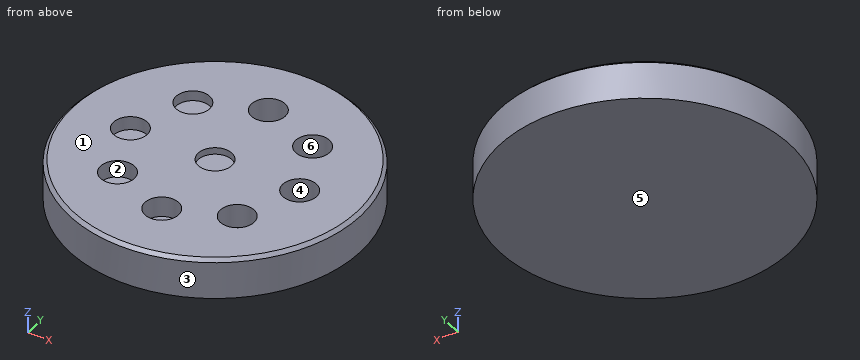
Autodesk Inventor part; units mm, degrees
ref_plane "YZ Plane" through (0, 0, 0) normal (1, 0, 0) x (0, 1, 0)
ref_plane "XZ Plane" through (0, 0, 0) normal (0, 1, 0) x (-1, 0, 0)
ref_plane "XY Plane" through (0, 0, 0) normal (0, 0, 1) x (1, 0, 0)
sketch "Sketch1" plane through (0, 0, 0) normal (0, 0, 1) x (1, 0, 0)
  circle A0 centre (0, 0) radius 43
  circle A1 centre (0, 0) radius 5
  circle A2 centre (0, 25) radius 5
  circle A3 centre (-17.6777, 17.6777) radius 5
  circle A4 centre (-25, 0) radius 5
  circle A5 centre (-17.6777, -17.6777) radius 5
  circle A6 centre (0, -25) radius 5
  circle A7 centre (17.6777, -17.6777) radius 5
  circle A8 centre (25, 0) radius 5
  circle A9 centre (17.6777, 17.6777) radius 5
  dimension "diameter" = 10
  dimension "d2" = 10
  dimension "d5" = 360
  dimension "d7" = 25
  dimension "d28" = 86
extrude "Extrusion1" add sketch "Sketch1" along normal blind 12
extrude "Extrusion2" add sketch "Sketch1" along normal blind 2 contours A2
extrude "Extrusion3" add sketch "Sketch1" along normal blind 3 contours A9
extrude "Extrusion4" add sketch "Sketch1" along normal blind 4 contours A8
extrude "Extrusion5" add sketch "Sketch1" along normal blind 5 contours A7
extrude "Extrusion6" add sketch "Sketch1" along normal blind 6 contours A6
extrude "Extrusion7" add sketch "Sketch1" along normal blind 7 contours A5
extrude "Extrusion8" add sketch "Sketch1" along normal blind 8 contours A4
extrude "Extrusion9" add sketch "Sketch1" along normal blind 9 contours A3
extrude "Extrusion10" add sketch "Sketch1" along normal blind 10 contours A1
sketch "Sketch2" plane through (0, 0, 12) normal (0, 0, 1) x (1, 0, 0)
  line L0 (-5.8774, 39.105) -> (5.7366, 39.105) construction
  line L1 (5.7366, 39.105) -> (5.7366, 35.936) construction
  line L2 (5.7366, 35.936) -> (-5.8774, 35.936) construction
  line L3 (-5.8774, 35.936) -> (-5.8774, 39.105) construction
  point P0 (0, 0)
emboss "Emboss1" [suppressed]
chamfer "Chamfer1" distance 1 angle 45 1 edges at (-43, 0, 12)
equation "\"d2\" = diameter"
properties part number "Diameter_10mm"
Can you work these out from the model? Positions are in its coordinate system, mm. Face numbers are marked on the shaded views. A direction names the side the tool comes from. Give positions to 0.01 mm unless a question says otherwise; leave off trailing zeros. Loops run counter-clockwise (first coordinate to the right, second up) from the corner with the lowest first, then second, coordinate; pieces in that order, holes last. Notation, with made-up numbers: M -2,54 L 43,54 A24 cw 43,67 Z; hole C 32.5,-31 d2. An arc over 180 degrees is marked long. One line per item, written item: value.
(1) Suppose I cut it at A-A on x = 0. List the corners of the cut face in (y, z) for me.
Returned:
outline: M -43,0 L 43,0 L 43,11 L 42,12 L 30,12 L 30,2 L 20,2 L 20,12 L 5,12 L 5,10 L -5,10 L -5,12 L -20,12 L -20,6 L -30,6 L -30,12 L -42,12 L -43,11 Z
(2) Suppose I cut it at B-B on y = 0. List the corners of the cut face in (x, z) for me.
Returned:
outline: M -43,0 L 43,0 L 43,11 L 42,12 L 30,12 L 30,4 L 20,4 L 20,12 L 5,12 L 5,10 L -5,10 L -5,12 L -20,12 L -20,8 L -30,8 L -30,12 L -42,12 L -43,11 Z
(3) I need wall thicknesses on line 1 (Y direction, x = 0, z = 5.75); line 2 (Y direction, x = 15, z = 7.75); line 3 (Y direction, x = 0, z = 11.1). Which ranges of each line are inside material? Lowest first, please.
Returned:
line 1: -43 to 20, 30 to 43
line 2: -40.3 to -21.9, -13.46 to 13.46, 21.9 to 40.3
line 3: -42.9 to -30, -20 to -5, 5 to 20, 30 to 42.9
(4) Which directions (+Z, -Z, +X, -X, +Y, -Y) give clear straight access to the entire face, cutting with the end or side of a thin tool? Please do the marked faces 5 and 6.
Returned:
face 5: -Z, +X, -X, +Y, -Y
face 6: +Z
(5) Will these pins go through, and if not, where does the flat tip stop? pin 1 (1 mm diameter, centred on y = 24.5, z = 9.5, fed in from +X); pin 2 (1.5 mm diameter, centred on x = -20, z = 5.5, fed in from +Y); pin 3 (1.5 mm diameter, centred on x = -11, z = 10.5, fed in from -Y).
Returned:
pin 1: x = 35.68
pin 2: y = 38.45
pin 3: y = -41.76
(6) We'd pull the mould along Y, two halves only. Please class the marked faces 1, 2, 3 and 4: released by +Y, released by -Y, zero draft, split by the parting line, or undercut.
Returned:
face 1: zero draft
face 2: undercut
face 3: split by the parting line
face 4: undercut
